Build history of the part. All positions in model axes, mm. A direction names the side the tool comes from. Coordinates: 2 decimals unless noted, no trailing zeros. Order: outer loops, then holes, each group sorted by start corner. A loop starts at its lowest first (then second) coordinate and runs counter-clockwise, first axis right, second up. Notation, with made-up numbers: M 21,35.5 L 50,35.5 A16 cw 50,41.5 Z; hole C 80,44.25 d3. An arc over 180 degrees is marked long. Use a Markdown table: item, result. Add a question column.
Autodesk Inventor part; units mm, degrees
ref_plane "YZ Plane" through (0, 0, 0) normal (1, 0, 0) x (0, 1, 0)
ref_plane "XZ Plane" through (0, 0, 0) normal (0, 1, 0) x (-1, 0, 0)
ref_plane "XY Plane" through (0, 0, 0) normal (0, 0, 1) x (1, 0, 0)
sketch "Sketch1" plane through (0, 0, 0) normal (0, 1, 0) x (-1, 0, 0)
  line L0 (-6.5, 22.5) -> (-6.5, -22.5)
  line L1 (-6.5, -22.5) -> (6.5, -22.5)
  line L2 (6.5, -22.5) -> (6.5, 22.5)
  line L3 (6.5, 22.5) -> (-6.5, 22.5)
  line L4 (-6.5, 22.5) -> (6.5, -22.5) construction
  line L5 (-6.5, -22.5) -> (6.5, 22.5) construction
  circle A0 centre (0, -22.5) radius 3
  circle A1 centre (0, -22.5) radius 6.5
  circle A2 centre (0, 22.5) radius 3
  circle A3 centre (0, 22.5) radius 6.5
  line L6 (-5, 16) -> (-5, -16)
  line L7 (-5, -16) -> (5, -16)
  line L8 (5, -16) -> (5, 16)
  line L9 (5, 16) -> (-5, 16)
  line L10 (-5, 16) -> (5, -16) construction
  line L11 (-5, -16) -> (5, 16) construction
  line L12 (-6.5, -16) -> (-6.5, -6)
  line L13 (-6.5, -6) -> (-16.5, -6)
  line L14 (-16.5, -6) -> (-16.5, -16)
  line L15 (-16.5, -16) -> (-6.5, -16)
  line L16 (-6.5, 16) -> (-6.5, 6)
  line L17 (-6.5, 6) -> (-16.5, 6)
  line L18 (-16.5, 6) -> (-16.5, 16)
  line L19 (-16.5, 16) -> (-6.5, 16)
  point P0 (0, 0)
  dimension "d0" = 45
  dimension "d1" = 13
  dimension "d2" = 6
  dimension "d3" = 6
  dimension "d4" = 10
  dimension "d5" = 10
  dimension "d6" = 10
  dimension "d7" = 10
  dimension "d8" = 10
extrude "Extrusion1" add sketch "Sketch1" along normal blind 5 contours A3 L9 L6 L7 A1 L0 | A3 L3 A2 | L3 A2 A3 | L2 A1 L7 L8 L9 A3 | A1 L1 A0 | L1 A0 A1
extrude "Extrusion2" add sketch "Sketch1" along normal blind 3 contours L0 L17 L18 L19 | L0 L15 L14 L13
extrude "Extrusion3" add sketch "Sketch1" along normal blind 16 contours L9 L8 L7 L6
sketch "Sketch2" plane through (-5, 5, 16) normal (0, 0, 1) x (1, 0, 0)
  line L0 (10, 11) -> (0, 11)
  line L1 (0, 11) -> (2, 11)
  line L2 (10, 0) -> (10, 11)
  line L3 (11.5, 0) -> (-1.5, 0)
  line L4 (0, 0) -> (0, 11)
  arc A0 (2, 11) -> (10, 3) centre (8.8459, 9.8459) ccw
  point P0 (5, -5)
  point P1 (3, 6.101)
  dimension "d15" = 2
  dimension "d16" = 3
  dimension "d17" = 5
  dimension "d18" = 3
extrude "Extrusion4" cut sketch "Sketch2" against normal through all contours L2 A0 L0
sketch "Sketch3" plane through (-5, 5, 16) normal (-1, 0, 0) x (0, 0, 1)
  line L0 (0, 11) -> (-32, 11)
  line L1 (-32, 11) -> (0, 11)
  line L2 (0, 0) -> (0, 11)
  line L3 (-38.5, 0) -> (6.5, 0)
  line L4 (-19, 11) -> (-19, 3)
  line L5 (-19, 3) -> (-32, 3)
  line L6 (-13, 11) -> (-13, 3)
  line L7 (-13, 3) -> (0, 3)
  line L8 (-32, 3) -> (-19, 3)
  line L9 (-19, 3) -> (-19, 11)
  line L10 (-19, 11) -> (-32, 11)
  line L11 (-32, 11) -> (-32, 3)
  line L12 (-13, 3) -> (0, 3)
  line L13 (0, 3) -> (0, 11)
  line L14 (0, 11) -> (-13, 11)
  line L15 (-13, 11) -> (-13, 3)
  line L16 (-21, 3) -> (-21, 11)
  line L17 (-11, 11) -> (-11, 3)
  point P0 (-16, -5)
  point P1 (-16, 11)
  point P2 (-16, 11)
  point P3 (-16, 11)
  point P4 (-11, 3)
  dimension "d21" = 3
  dimension "d22" = 3
  dimension "d23" = 3
  dimension "d24" = 3
  dimension "d25" = 32
  dimension "d26" = 2
  dimension "d27" = 2
extrude "Extrusion5" cut sketch "Sketch3" against normal blind 10 contours L4 L5 L16 L0 | L17 L7 L6 L0
chamfer "Chamfer1" distance 2 angle 45 2 edges at (3, 5, -22.5) (3, 5, 22.5)
properties part number "string_holderWPNB"
(1) Which spindle directions (+Z, -Z, +X, -X, +Y, -Y) get a long thin tool onto all of the face, cutting with end or side? Do faces 1 (the flat face through (-1, 8, -4)), 2 (the flat face through (5, 6, 0)), 3 (the flat face through (-1, 8, 16)). Say none if no direction does.
(2) Mould opens along Y. For faces 4 (the cylindrical face through (-1.128, 10.003, 0.224)), 5 (the flat face through (-3, 11, -5)), 6 (the flat face through (-4, 16, 0)) say: released by +Y, released by -Y, zero draft, split by the parting line, or undercut.
(3) Slice it at D-D on x = 0. Give the cut face in (y, z).
(4) Slice it at C-C on y = 2. Give the cut face in (x, z).
(5) Slice it at B-B on z = -1.5. Give the cut face in (x, y) (1 decimal), and give its area (3 significant figures).
(6) Slice it at A-A on x = 9. Give the cut face in (y, z), and give its area (3 significant figures).
(7) Drill centre lines: line 1 along Z through (x, y) = (0, 1.55); line 2 along X through (y, z) = (2, 22.5); line 3 along Z through (x, y) = (-2.25, 11.25). Where is each one in solid material? Low to high. Write a range as from..to.
(8) Drop flat-ended pins along their axis: P1, Ø3, axis at x = 5.5, z = 8.5, coming from the -Y side; P2, Ø8, axis at x = 1.5, y = 10, coming from the -Z side; P3, Ø6, axis at x = -2, y = 12.5, coming from the +Z side; P4, Ø4, axis at x = 1, z = -3.5, coming from the +Y side. Give the stop position or say it passes through.
Solutions:
| question | item | result |
|---|---|---|
| 1 | face 1 | +X, -X, +Y |
| 1 | face 2 | +Z, -Z, +X, +Y |
| 1 | face 3 | +Z, +X, -X, +Y |
| 2 | face 4 | undercut |
| 2 | face 5 | zero draft |
| 2 | face 6 | released by +Y |
| 3 | outline | M 0,-29 L 5,-29 L 5,-27.5 L 3,-25.5 L 0,-25.5 Z; M 0,-19.5 L 3,-19.5 L 5,-17.5 L 5,-16 L 9.07,-16 L 9.07,-5 L 8,-5 L 8,-3 L 9.07,-3 L 9.07,3 L 8,3 L 8,5 L 9.07,5 L 9.07,16 L 5,16 L 5,17.5 L 3,19.5 L 0,19.5 Z; M 0,25.5 L 3,25.5 L 5,27.5 L 5,29 L 0,29 Z |
| 4 | outline | M -6.5,-22.5 A6.5 ccw 6.5,-22.5 L 6.5,-16 L 16.5,-16 L 16.5,-6 L 6.5,-6 L 6.5,6 L 16.5,6 L 16.5,16 L 6.5,16 L 6.5,22.5 A6.5 ccw -6.5,22.5 Z; hole C 0,-22.5 d6; hole C 0,22.5 d6 |
| 5 | outline | M -6.5,0 L 6.5,0 L 6.5,5 L 5,5 L 5,8 A6.9 cw -3,16 L -5,16 L -5,5 L -6.5,5 Z |
| 5 | area | 120 mm² |
| 6 | outline | M 0,-16 L 3,-16 L 3,-6 L 0,-6 Z; M 0,6 L 3,6 L 3,16 L 0,16 Z |
| 6 | area | 60.0 mm² |
| 7 | line 1 | -29..-25.5, -19.5..19.5, 25.5..29 |
| 7 | line 2 | -6.5..-3, 3..6.5 |
| 7 | line 3 | -16..-5, -3..3, 5..16 |
| 8 | P1 | y = 0 |
| 8 | P2 | z = -16 |
| 8 | P3 | z = 16 |
| 8 | P4 | y = 9.81 |
